The model under review builds one solid part; all positions refer to its coordinate system, in mm. A direction names the side the tool comes from. Round coordinates to 2 decimals unless told otherwise and drop trailing zeros. Loops run counter-clockwise (first coordinate to the right, second up) from the corner with the lowest first, then second, coordinate; pieces in that order, holes last. Notation, with made-up numbers: M 28.5,29.25 L 85.5,29.25 A33 cw 85.5,65.25 Z; hole C 22.25,29 d10. An arc over 180 degrees is marked long. One line per question, with ' | ' between items.
from build123d import *

# Parameters (mm, degrees)
PAD_DEPTH    = 20
SKETCH001_R  = 4
POCKET_DEPTH = 25.001
CHAMFER_SIZE = 2


with BuildPart() as part:
    # Sketch → Pad (new body, symmetric)
    with BuildSketch(Plane.XY):
        with BuildLine():
            Line((-40, 0), (-20, 0))
            ThreePointArc((20, 0), (0, 20), (-20, 0))
            Line((20, 0), (40, 0))
            Line((40, -5), (40, 0))
            Line((15, -5), (40, -5))
            Line((15, 0), (15, -5))
            ThreePointArc((15, 0), (0, 15), (-15, 0))
            Line((-15, 0), (-15, -5))
            Line((-15, -5), (-40, -5))
            Line((-40, -5), (-40, 0))
        make_face()
    extrude(amount=PAD_DEPTH, both=True)

    # Sketch001 → Pocket (cut, through all)
    with BuildSketch(Plane.XZ.offset(5)):
        with Locations((-30, 0)):
            Circle(SKETCH001_R)
        with Locations((30, 0)):
            Circle(SKETCH001_R)
    extrude(amount=-POCKET_DEPTH, mode=Mode.SUBTRACT)

    # Chamfer
    chamfer_edges = [part.edges().sort_by_distance(p)[0] for p in [
        (26, 0, 0),
        (-34, 0, 0),
    ]]
    chamfer(chamfer_edges, length=CHAMFER_SIZE)


solid = part.part
1) Add section B-B on x = -30. State the section outline as (y, z) points, then the cut area to 3 significant figures.
Output values:
outline: M -5,-20 L 0,-20 L 0,-6 L -2,-4 L -5,-4 Z; M -5,4 L -2,4 L 0,6 L 0,20 L -5,20 Z | area: 156 mm²
2) Add section C-C on z = 0. State the section outline as (x, y) points, then the cut area to 3 significant figures.
Output values:
outline: M -40,-5 L -34,-5 L -34,-2 L -36,0 L -40,0 Z; M -26,-5 L -15,-5 L -15,0 A15 cw 15,0 L 15,-5 L 26,-5 L 26,-2 L 24,0 L 20,0 A20 ccw -20,0 L -24,0 L -26,-2 Z; M 34,-5 L 40,-5 L 40,0 L 36,0 L 34,-2 Z | area: 437 mm²
3) Add section D-D on y = 5.5. State the section outline as (x, z) points.
Output values:
outline: M -19.23,-20 L -13.96,-20 L -13.96,20 L -19.23,20 Z; M 13.96,-20 L 19.23,-20 L 19.23,20 L 13.96,20 Z
4) Machinability: for faces 4 (the flat face through (-15, -2, 0)), 5 (the flat face through (25, 0, 5)), 6 (the flat face through (-35, 0, 5)), which of the approach directions +Z, -Z, +X, -X, +Y, -Y give a long, thin tool a straight path to every point of the face, cutting with its end or side? Answer none if there is none.
Output values:
face 4: +Z, -Z, -Y | face 5: +Z, -Z, +X, +Y | face 6: +Z, -Z, -X, +Y
5) Mouldability with a two-part tool opening along Z and no side actions: class faces 1 (the flat face through (9.1, 12.2, 20)), 2 (the cylindrical face through (-33.2, -3.5, -2.4)), 3 (the flat face through (15, -2, 0)) as +Z half, -Z half, draft (parallel to the pull), parting line (faces both ways), or undercut.
Output values:
face 1: +Z half | face 2: undercut | face 3: draft
6) For line 1 (Y direction, x = 23, z = -17.5); line 2 (X direction, y = 8.5, z = -16); line 3 (Z direction, x = -30, y = -4), list the stretches that pass through material, from the lowest coordinate up.
Output values:
line 1: y = -5 to 0 | line 2: x = -18.1 to -12.36, 12.36 to 18.1 | line 3: z = -20 to -4, 4 to 20
7) Add section A-A on y = -1. State the section outline as (x, z) points, then the cut area to 3 significant figures.
Output values:
outline: M -40,-20 L -15,-20 L -15,20 L -40,20 Z; M 15,-20 L 40,-20 L 40,20 L 15,20 Z; hole C -30,0 d10; hole C 30,0 d10 | area: 1,840 mm²
8) Insertion check: P1, Ø6, axis at x = -17.5, z = 9.5, coming from the +Y side (3 decimals); P2, Ø8, axis at x = 8.5, z = -8, coming from the -Y side; P3, Ø6, axis at x = -31.5, z = -2, coming from the +Y side. Each pin has a flat end and moves straight along its axis. Give the tip position at first contact, or say it passes through.
Output values:
P1: stops at y = 13.775 | P2: stops at y = 8.29 | P3: stops at y = -0.5
